Part model, mm, in its own coordinate system. A direction names the side the tool comes from. Round coordinates to 2 decimals unless told otherwise and drop trailing zeros. Order: outer loops, then holes, each group sorted by start corner. A loop starts at its lowest first (then second) coordinate and runs counter-clockwise, first axis right, second up. Notation, with made-up numbers: M 12.5,40.25 L 38.5,40.25 A6 ccw 38.5,49.25 Z; hole C 75,-40 d5. An arc over 180 degrees is marked long. Write each question's results on one line, items separated by ' | '. Start each with the question number.
1. Which spindle directions (+Z, -Z, +X, -X, +Y, -Y) get a long thin tool onto all of the face, cutting with end or side? Do faces 4 (the face through (-95, 0, 80)), 5 (the face through (59, 62, 30)), 6 (the face through (-3.252, -74.643, 50.14)), 7 (the face through (6, -20, 90)), 8 (the face through (5.42, -84.406, 9.86)). Say none if no direction does.
2. Band-saw the part on D-D, the plane z = 35. List the corners of the cut face in (x, y), then the cut area to 3 significant figures.
3. Band-saw the part on B-B, the plane y = 55. List the corners of the cut face in (x, z), then the cut area to 3 significant figures.
4. Band-saw the part on C-C, the plane x = -12.5. List the corners of the cut face in (y, z), then the cut area to 3 significant figures.
5. Drop flat-ended pins along their axis: pin 1 Ø3 at (x, z) = (-49.5, 77.5) entering from +Y; pin 2 Ø12 at (x, z) = (77.5, 72) entering from +Y; pin 3 Ø6 at (x, z) = (55, 65.5) entering from -Y. Give the stop position or say it passes through.
6. Band-saw the part on A-A, the plane z = 63.5. List the corners of the cut face in (x, y), then the cut area to 3 significant figures.
7. Probe L1, parallel to Y at x = 0, z = 55.5; L2, parallel to Y at x = 12, z = 62.5; L3, parallel to X at y = -15.5, z = 81.5. List the from-to ranges inside material, lowest first. Write a range as [from, to].
8. Two-plate mould, pull along Y, no slides. Class faces 1 (the face through (-13.02, -99.15, 38.19)), 2 (the face through (-1, -36, 60)), 3 (the face through (-68, 60, 30)): +Y half, -Y half, draft (parallel to the pull), parting line (faces both ways), or undercut.
```python
from build123d import *

# Parameters (mm, degrees)
SKETCH1_R           = 100
BOSS_EXTRUDE1_DEPTH = 100
SKETCH3_R           = 7.5
CUT_EXTRUDE2_DEPTH  = 30
CUT_EXTRUDE3_DEPTH  = 70
SKETCH5_W           = 200
SKETCH5_H           = 200
CUT_EXTRUDE4_DEPTH  = 70
BOSS_EXTRUDE2_DEPTH = 40
SKETCH7_R           = 15
CUT_EXTRUDE5_DEPTH  = 20
SKETCH8_R           = 5
CUT_EXTRUDE6_DEPTH  = 89
SKETCH9_R           = 25
CUT_EXTRUDE7_DEPTH  = 20
SKETCH10_R          = 30
BOSS_EXTRUDE4_DEPTH = 30
SKETCH12_R          = 20
CUT_EXTRUDE9_DEPTH  = 50
SKETCH13_R          = 20
CUT_EXTRUDE10_DEPTH = 50


with BuildPart() as part:
    # Sketch1 → Boss-Extrude1 (new body)
    with BuildSketch(Plane.XY):
        Circle(SKETCH1_R)
    extrude(amount=BOSS_EXTRUDE1_DEPTH)

    # Sketch3 → Cut-Extrude2 (cut)
    with BuildSketch(Plane(origin=(0, 0, 0), x_dir=(-1, 0, 0), z_dir=(0, 0, -1))):
        with Locations((-55, 55)):
            Circle(SKETCH3_R)
        with Locations((55, 55)):
            Circle(SKETCH3_R)
    extrude(amount=-CUT_EXTRUDE2_DEPTH, mode=Mode.SUBTRACT)

    # Sketch4 → Cut-Extrude3 (cut)
    with BuildSketch(Plane.XY.offset(100)):
        with BuildLine():
            ThreePointArc((-97.979589711, 20), (-48.511807343, 48.511807343), (-20, 97.979589711))
            ThreePointArc((-20, 97.979589711), (-70.710678119, 70.710678119), (-97.979589711, 20))
        make_face()
        with BuildLine():
            ThreePointArc((97.979589711, 20), (70.710678119, 70.710678119), (20, 97.979589711))
            ThreePointArc((20, 97.979589711), (48.511807343, 48.511807343), (97.979589711, 20))
        make_face()
    extrude(amount=-CUT_EXTRUDE3_DEPTH, mode=Mode.SUBTRACT)

    # Sketch5 → Cut-Extrude4 (cut)
    with BuildSketch(Plane.XY.offset(60)):
        Rectangle(SKETCH5_W, SKETCH5_H)
    extrude(amount=CUT_EXTRUDE4_DEPTH, mode=Mode.SUBTRACT)

    # Sketch6 → Boss-Extrude2 (add)
    with BuildSketch(Plane.XY.offset(60)):
        with BuildLine():
            Line((-100, 0), (-90, 0))
            ThreePointArc((-90, 0), (0, -90), (90, 0))
            Line((90, 0), (100, 0))
            ThreePointArc((100, 0), (0, -100), (-100, 0))
        make_face()
    extrude(amount=BOSS_EXTRUDE2_DEPTH)

    # Sketch7 → Cut-Extrude5 (cut)
    with BuildSketch(Plane.XY.offset(60)):
        with Locations((0, -60)):
            Circle(SKETCH7_R)
    extrude(amount=-CUT_EXTRUDE5_DEPTH, mode=Mode.SUBTRACT)

    # Sketch8 → Cut-Extrude6 (cut)
    with BuildSketch(Plane.XY.offset(40)):
        with Locations((0, -60)):
            Circle(SKETCH8_R)
    extrude(amount=-CUT_EXTRUDE6_DEPTH, mode=Mode.SUBTRACT)

    # Sketch9 → Cut-Extrude7 (cut)
    with BuildSketch(Plane(origin=(0, 0, 0), x_dir=(-1, 0, 0), z_dir=(0, 0, -1))):
        with Locations((0, -60)):
            Circle(SKETCH9_R)
    extrude(amount=-CUT_EXTRUDE7_DEPTH, mode=Mode.SUBTRACT)

    # Sketch10 → Boss-Extrude4 (add)
    with BuildSketch(Plane.XY.offset(60)):
        Circle(SKETCH10_R)
    extrude(amount=BOSS_EXTRUDE4_DEPTH)

    # Sketch12 → Cut-Extrude9 (cut)
    with BuildSketch(Plane.XY.offset(90)):
        Circle(SKETCH12_R)
    extrude(amount=-CUT_EXTRUDE9_DEPTH, mode=Mode.SUBTRACT)

    # Sketch13 → Cut-Extrude10 (cut)
    with BuildSketch(Plane.XY.offset(40)):
        Circle(SKETCH13_R)
    extrude(amount=-CUT_EXTRUDE10_DEPTH, mode=Mode.SUBTRACT)


solid = part.part
```
Solution:
1) face 4: +Z, -X, +Y | face 5: +Z, +X, +Y | face 6: +Z | face 7: +Z, +Y | face 8: -Z
2) outline: M -97.98,20 A100 ccw long 97.98,20 A110 cw 20,97.98 A100 ccw -20,97.98 A110 cw Z; hole C 0,0 d40; hole C 0,-60 d10 | area: 25,400 mm^2
3) outline: M -83.52,0 L -62.5,0 L -62.5,30 L -83.52,30 Z; M -47.5,0 L 47.5,0 L 47.5,30 L 42.52,30 L 42.52,60 L -42.52,60 L -42.52,30 L -47.5,30 Z; M 62.5,0 L 83.52,0 L 83.52,30 L 62.5,30 Z | area: 6,660 mm^2
4) outline: M -99.22,0 L -81.65,0 L -81.65,20 L -38.35,20 L -38.35,0 L -15.61,0 L -15.61,90 L -27.27,90 L -27.27,60 L -51.71,60 L -51.71,40 L -68.29,40 L -68.29,60 L -89.13,60 L -89.13,100 L -99.22,100 Z; M 15.61,0 L 99.22,0 L 99.22,60 L 27.27,60 L 27.27,90 L 15.61,90 Z | area: 9,940 mm^2
5) pin 1: y = -74.16 | pin 2: y = -33.58 | pin 3: y = -85.42
6) outline: M -100,0 A100 ccw 100,0 L 90,0 A90 cw -90,0 Z; C 0,0 d60; hole C 0,0 d40 | area: 4,560 mm^2
7) L1: [-100, -75], [-45, -20], [20, 100] | L2: [-99.28, -89.2], [-27.5, -16], [16, 27.5] | L3: [-98.79, -88.66], [-25.69, -12.64], [12.64, 25.69], [88.66, 98.79]
8) face 1: parting line | face 2: undercut | face 3: draft
